Source: three-view drawing plus pictorial views. Frame: mm from the lowest corner of the part. Give positions to 0.01 mm unless a question says otherwise; leave off trailing zeros. Write each loop counter-clockwise with the first axis right and the second up, starting at its lowest first coordinate (ties: lowest second). Pieces come first, ordered by that corner, then holes. Notation, with made-up numbers: (36.25, 48) - (42.25, 48) arc R7 cw to (42.25, 60) - close; hole circle Ø5 at (73.25, -27). An arc over 180 degrees is marked (long way). One line per question, with ' | ' between items. Start each with the question number.
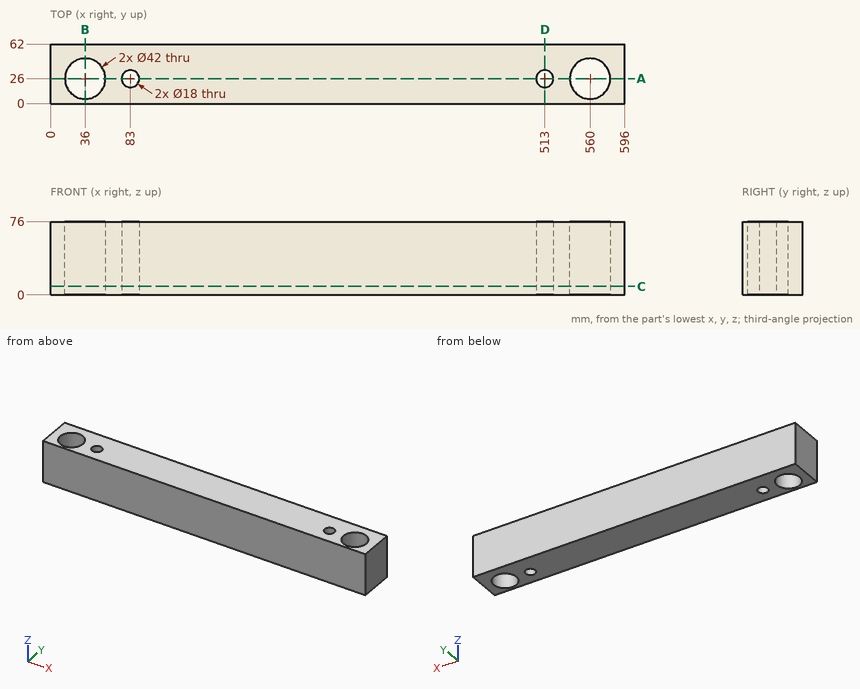
1) Section A-A, the plane y = 26. Output: boundary loops of the cut face in (x, z).
2) Section D-D, the plane x = 513. Output: boundary loops of the cut face in (y, z), plus the area to 3 significant figures.
3) Section B-B, the plane x = 36. Output: boundary loops of the cut face in (y, z), plus the area to 3 significant figures.
4) Section C-C, the plane z = 9. Output: boundary loops of the cut face in (x, y), plus the area to 3 significant figures.
5) First-contact query: pin 1 Ø8 at (y, z) = (55.5, 9.5) entering from -X. Flat tip, straight axial feed; report the tip coordinate or a pass-through.
6) Line query: L1, parallel to Y at x = 514, z = 42; L2, parallel to Y at x = 513, z = 50.5; L3, parallel to X at y = 18.5, z = 66. Output: solid intervals per line, ascending.
Answer key:
1) outline: (0, 0) - (15, 0) - (15, 76) - (0, 76) - close; (57, 0) - (74, 0) - (74, 76) - (57, 76) - close; (92, 0) - (504, 0) - (504, 76) - (92, 76) - close; (522, 0) - (539, 0) - (539, 76) - (522, 76) - close; (581, 0) - (596, 0) - (596, 76) - (581, 76) - close
2) outline: (0, 0) - (17, 0) - (17, 76) - (0, 76) - close; (35, 0) - (62, 0) - (62, 76) - (35, 76) - close | area: 3,340 mm^2
3) outline: (0, 0) - (5, 0) - (5, 76) - (0, 76) - close; (47, 0) - (62, 0) - (62, 76) - (47, 76) - close | area: 1,520 mm^2
4) outline: (0, 0) - (596, 0) - (596, 62) - (0, 62) - close; hole circle Ø42 at (36, 26); hole circle Ø18 at (83, 26); hole circle Ø18 at (513, 26); hole circle Ø42 at (560, 26) | area: 33,700 mm^2
5) pin 1: x = 0
6) L1: 0 to 17.06, 34.94 to 62 | L2: 0 to 17, 35 to 62 | L3: 0 to 16.38, 55.62 to 78.03, 87.97 to 508.03, 517.97 to 540.38, 579.62 to 596
